```python
from build123d import *

# Parameters (mm, degrees)
EXTRUDE_1_DEPTH     = 20
EXTRUDE_2_DEPTH     = 2
CUT_EXTRUDE_2_DEPTH = 30
CUT_EXTRUDE_3_DEPTH = 30
SKETCH_8_W          = 27
SKETCH_8_H          = 18
SKETCH_8_R          = 5
EXTRUDE_3_DEPTH     = 3
SKETCH_9_W          = 24
SKETCH_9_H          = 18
SKETCH_9_R          = 5
EXTRUDE_4_DEPTH     = 3
CUT_EXTRUDE_4_DEPTH = 30
SKETCH_12_W         = 30
SKETCH_12_H         = 3.25
CUT_EXTRUDE_5_DEPTH = 30
EXTRUDE_5_DEPTH     = 3


with BuildPart() as part:
    # 草图1 → 凸台-拉伸1 (new body)
    with BuildSketch(Plane(origin=(0, 0, 0), x_dir=(1, 0, 0), z_dir=(0, 1, 0))):
        Polygon((0, 0), (0, 30), (3, 30), (3, 3), (30, 3), (30, 0), align=None)
    extrude(amount=EXTRUDE_1_DEPTH)

    # 草图2 → 凸台-拉伸2 (add)
    with BuildSketch(Plane.XZ):
        Polygon((3, -30), (30, -3), (3, -3), align=None)
    extrude(amount=-EXTRUDE_2_DEPTH)

    # 草图5 → 切除-拉伸2 (cut)
    with BuildSketch(Plane(origin=(0, 0, -3), x_dir=(-1, 0, 0), z_dir=(0, 0, -1))):
        with BuildLine():
            ThreePointArc((-13.9, 10), (-15.685152354, 12.469012619), (-18.589248703, 11.547591632))
            Line((-18.589248703, 11.547591632), (-14.410751297, 8.452408368))
            ThreePointArc((-14.410751297, 8.452408368), (-14.030987381, 9.185152354), (-13.9, 10))
        make_face()
        with BuildLine():
            Line((-14.410751297, 8.452408368), (-18.589248703, 11.547591632))
            ThreePointArc((-18.589248703, 11.547591632), (-18.047591632, 7.910751297), (-14.410751297, 8.452408368))
        make_face()
    extrude(amount=-CUT_EXTRUDE_2_DEPTH, mode=Mode.SUBTRACT)

    # 草图7 → 切除-拉伸3 (cut)
    with BuildSketch(Plane(origin=(3, 0, 0), x_dir=(0, 0, -1), z_dir=(1, 0, 0))):
        with BuildLine():
            ThreePointArc((19.1, 10), (17.314847646, 12.469012619), (14.410751297, 11.547591632))
            Line((14.410751297, 11.547591632), (18.589248703, 8.452408368))
            ThreePointArc((18.589248703, 8.452408368), (18.969012619, 9.185152354), (19.1, 10))
        make_face()
        with BuildLine():
            Line((18.589248703, 8.452408368), (14.410751297, 11.547591632))
            ThreePointArc((14.410751297, 11.547591632), (14.952408368, 7.910751297), (18.589248703, 8.452408368))
        make_face()
    extrude(amount=-CUT_EXTRUDE_3_DEPTH, mode=Mode.SUBTRACT)

    # 草图8 → 凸台-拉伸3 (add)
    with BuildSketch(Plane(origin=(0, 0, -3), x_dir=(-1, 0, 0), z_dir=(0, 0, -1))):
        with Locations((-16.5, 11)):
            Rectangle(SKETCH_8_W, SKETCH_8_H)
        with Locations((-16.5, 10)):
            Circle(SKETCH_8_R, mode=Mode.SUBTRACT)
    extrude(amount=EXTRUDE_3_DEPTH)

    # 草图9 → 凸台-拉伸4 (add)
    with BuildSketch(Plane(origin=(3, 0, 0), x_dir=(0, 0, -1), z_dir=(1, 0, 0))):
        with Locations((18, 11)):
            Rectangle(SKETCH_9_W, SKETCH_9_H)
        with Locations((16.5, 10)):
            Circle(SKETCH_9_R, mode=Mode.SUBTRACT)
    extrude(amount=EXTRUDE_4_DEPTH)

    # 草图10 → 切除-拉伸4 (cut)
    with BuildSketch(Plane.XZ.offset(-2)):
        Polygon((3, -30), (6, -27), (6, -30), align=None)
        Polygon((27, -6), (30, -3), (30, -6), align=None)
    extrude(amount=-CUT_EXTRUDE_4_DEPTH, mode=Mode.SUBTRACT)

    # 草图12 → 切除-拉伸5 (cut)
    with BuildSketch(Plane(origin=(30, 0, 0), x_dir=(0, 0, -1), z_dir=(1, 0, 0))):
        with Locations((15, 18.375)):
            Rectangle(SKETCH_12_W, SKETCH_12_H)
    extrude(amount=-CUT_EXTRUDE_5_DEPTH, mode=Mode.SUBTRACT)

    # 草图13 → 凸台-拉伸5 (add)
    with BuildSketch(Plane.XZ):
        Polygon((3, -30), (3, -3), (30, -3), align=None)
    extrude(amount=-EXTRUDE_5_DEPTH)


solid = part.part
```
Geometry check sheet. Reference: the model listing, model coordinates, mm. A direction names the side the tool comes from. Round coordinates to 2 decimals unless told otherwise and drop trailing zeros. Order: outer loops, then holes, each group sorted by start corner. A loop starts at its lowest first (then second) coordinate and runs counter-clockwise, first axis right, second up. Notation, with made-up numbers: (72.25, -32.5) -> (99.25, -32.5) arc R22 cw to (99.25, 4.5) -> close; hole circle Ø5 at (-37, 87.25). An arc over 180 degrees is marked (long way). Return JSON: item names as keys, results as strings. Group by question number.
Q1. Section check C-C, the plane y = 9.5. Record the boundary of the cut face in (x, z), plus the area to 3 significant figures.
Q2. Section check B-B, the plane z = -16.5. Record the boundary of the cut face in (x, y), plus the area to 3 significant figures.
Q3. Material ranges on probe 1 along Y at (x, z) = (4.85, -16.5); probe 2 along X at (y, z) = (10, -24.5); probe 3 along Z at (x, y) = (15, 7), recorded low to high. Write a range as from..to.
Q4. Gauge pin test, flat ends, axial feed: pin 1 (3 mm diameter, centred on x = 17.5, y = 10, fed in from -Z); pin 2 (4 mm diameter, centred on x = 19.5, y = 8, fed in from -Z); pin 3 (7 mm diameter, centred on y = 7.5, z = -12, fed in from +X); pin 4 (1.5 mm diameter, centred on y = 14.5, z = -5, fed in from +X). Record the tip position at first contact, or that the pin passes through.
Q5. Tool access check on faces 1 (the flat face through (6, 15, -14)), 2 (the flat face through (19, 12, -3)), 3 (the cylindrical face through (4.48, 11.5, -21.27)). Record the directions out of +Z, -Z, +X, -X, +Y, -Y that give a thin tool (end or side, any length) a straight path to the whole face; none if there is none.
Q6. Section check A-A, the plane x = 16.5. Record the boundary of the cut face in (y, z).
Q7. Section check D-D, the plane z = -12.5. Record the boundary of the cut face in (x, y), plus the area to 3 significant figures.
Q8. Release check for a two-part mould opening along Y. For faces 4 (the flat face through (3, 12, -14)), 5 (the flat face through (19, 15, -6)), 6 (the flat face through (12, 3, -12)) record: released by +Y, released by -Y, zero draft, split by the parting line, or undercut.
Numbers:
{
 "1": {"outline": "(0, -30) -> (3, -30) -> (6, -27) -> (6, -21.47) -> (3, -21.47) -> (3, -19.05) -> (0, -19.05) -> close; (0, -13.95) -> (3, -13.95) -> (3, -11.53) -> (6, -11.53) -> (6, -6) -> (11.53, -6) -> (11.53, -3) -> (13.95, -3) -> (13.95, 0) -> (0, 0) -> close; (19.05, -3) -> (21.47, -3) -> (21.47, -6) -> (27, -6) -> (30, -3) -> (30, 0) -> (19.05, 0) -> close", "area": "225 mm^2"},
 "2": {"outline": "(0, 0) -> (16.5, 0) -> (16.5, 3) -> (6, 3) -> (6, 5) -> (3, 5) -> (3, 7.4) -> (0, 7.4) -> close; (0, 12.6) -> (3, 12.6) -> (3, 15) -> (6, 15) -> (6, 16.75) -> (0, 16.75) -> close", "area": "86.4 mm^2"},
 "3": {"probe 1": "0..5, 15..16.75", "probe 2": "0..6", "probe 3": "-3..0"},
 "4": {"pin 1": "through", "pin 2": "z = -6", "pin 3": "x = 6", "pin 4": "x = 28.75"},
 "5": {"face 1": "-Z, +X, +Y", "face 2": "-Z", "face 3": "+X"},
 "6": {"outline": "(0, -16.5) -> (3, -16.5) -> (3, -6) -> (5, -6) -> (5, -3) -> (7.4, -3) -> (7.4, 0) -> (0, 0) -> close; (12.6, -3) -> (15, -3) -> (15, -6) -> (16.75, -6) -> (16.75, 0) -> (12.6, 0) -> close"},
 "7": {"outline": "(0, 0) -> (20.5, 0) -> (20.5, 3) -> (6, 3) -> (6, 7) -> (3, 7) -> (3, 13) -> (6, 13) -> (6, 16.75) -> (0, 16.75) -> close", "area": "126 mm^2"},
 "8": {"face 4": "undercut", "face 5": "zero draft", "face 6": "released by +Y"}
}
